For this review, take the finished solid that the model builds, in its own axes (mm). Coordinates: 2 decimals unless noted, no trailing zeros. Write each loop counter-clockwise with the first axis right and the second up, starting at its lowest first coordinate (ties: lowest second). Pieces come first, ordered by that corner, then holes.
1) Insertion check: P1, Ø1, axis at x = 291.5, z = -52.5, coming from the -Y side; P2, Ø12, axis at x = 464, y = -43.5, coming from the +Z side; P3, Ø5, axis at x = 453, z = -33, coming from the -Y side. Each pin has a flat end and moves straight along its axis. Give the tip position at first contact, or say it passes through.
2) We need section C-C on z = -54.5. Write out the cut boundary in (x, y), then the cut area to 3 significant figures.
3) We need section A-A on x = 116. Write out the cut boundary in (y, z), then the cut area to 3 significant figures.
4) Mouldability with a two-part tool opening along Z and no side actions: class faces 1 (the face through (900, -41, 65)), 2 (the face through (456.3, -23.73, 75.35)), 3 (the face through (456.3, 74.476, -16.538)) as pulls with the +Z half, pulls with the -Z half, needs draft (parallel to the pull), parting line crosses it, or undercut.
5) We need section B-B on y = 0. Write out the cut boundary in (x, z).
6) To check wall thickness, follow line 1 along Y through (x, z) = (185.5, 0); line 2 along Y through (x, z) = (89.5, 25); line 3 along Z through (x, y) = (788, -62). State the ranges of each line that lie inside material, in increasing order.
7) We need section D-D on x = 493. Write out the cut boundary in (y, z), then the cut area to 3 significant figures.
from build123d import *

# Parameters (mm, degrees)
ESQUISSE1_W                  = 900
ESQUISSE1_H                  = 2.71
ESQUISSE2_W                  = 150
ESQUISSE2_H                  = 3
ENL_V_MAT_EXTRU_1_DEPTH      = 907.907933585
R_P_TITION_CIRCULAIRE1_COUNT = 3
R_P_TITION_CIRCULAIRE1_ANGLE = 240


with BuildPart() as part:
    # Esquisse1 → Révolution1 (revolve)
    with BuildSketch(Plane.XY, mode=Mode.PRIVATE) as r_volution1_sk:
        with Locations((450, 77.645)):
            Rectangle(ESQUISSE1_W, ESQUISSE1_H)
    revolve(r_volution1_sk.sketch.rotate(Axis((0, 0, 0), (1, 0, 0)), 90), axis=Axis((0, 0, 0), (1, 0, 0)))

    # Esquisse2 → Enlèv. mat.-Extru.1 (cut, through all)
    with BuildSketch(Plane(origin=(0, 0, 0), x_dir=(1, 0, 0), z_dir=(0, 1, 0))):
        with Locations((75, 0)):
            Rectangle(ESQUISSE2_W, ESQUISSE2_H)
    enl_v_mat_extru_1 = extrude(amount=ENL_V_MAT_EXTRU_1_DEPTH, mode=Mode.SUBTRACT)

    # Répétition circulaire1: Enlèv. mat.-Extru.1 ×3 about axis
    r_p_tition_circulaire1_axis = Axis((0, 0, 0), (-1, 0, 0))
    for i in range(1, R_P_TITION_CIRCULAIRE1_COUNT):
        add(enl_v_mat_extru_1.rotate(r_p_tition_circulaire1_axis, i * R_P_TITION_CIRCULAIRE1_ANGLE / (R_P_TITION_CIRCULAIRE1_COUNT - 1)), mode=Mode.SUBTRACT)


solid = part.part
Result:
1. P1: stops at y = -59.47
1. P2: stops at z = 69.53
1. P3: stops at y = -72.87
2. outline: (0, -57.19) - (900, -57.19) - (900, -53.38) - (0, -53.38) - close; (0, 53.38) - (900, 53.38) - (900, 57.19) - (0, 57.19) - close
2. area: 6,850 mm2
3. outline: (-40.79, -67.65) - (-39.44, -65.31) arc R76.29 cw to (-39.44, 65.31) - (-40.79, 67.65) arc R79 ccw to start; (-38.19, -69.15) arc R79 ccw to (78.99, -1.5) - (76.28, -1.5) arc R76.29 cw to (-36.84, -66.81) - close; (-38.19, 69.15) - (-36.84, 66.81) arc R76.29 cw to (76.28, 1.5) - (78.99, 1.5) arc R79 ccw to start
3. area: 1,300 mm2
4. face 1: needs draft
4. face 2: parting line crosses it
4. face 3: undercut
5. outline: (0, -79) - (900, -79) - (900, -76.29) - (0, -76.29) - close; (0, 76.29) - (900, 76.29) - (900, 79) - (0, 79) - close
6. line 1: y = -79 to -76.29, 76.29 to 79
6. line 2: y = -74.94 to -72.08, 72.08 to 74.94
6. line 3: z = -48.96 to -44.45, 44.45 to 48.96
7. outline: circle Ø158 at (0, 0); hole circle Ø152.58 at (0, 0)
7. area: 1,320 mm2
